from build123d import *

# Parameters (mm, degrees)
SKETCH1_R             = 11
BOSS_EXTRUDE1_DEPTH   = 3
SKETCH1_3_R           = 11
CUT_EXTRUDE1_DEPTH    = 1
SKETCH2_W             = 3
SKETCH2_H             = 6
BOSS_EXTRUDE2_DEPTH   = 3
BOSS_EXTRUDE2_2_DEPTH = 3
SKETCH2_H_2           = 5.08
BOSS_EXTRUDE2_3_DEPTH = 3
BOSS_EXTRUDE2_4_DEPTH = 3
BOSS_EXTRUDE2_5_DEPTH = 3
SKETCH3_W             = 3
SKETCH3_H             = 3
CUT_EXTRUDE2_DEPTH    = 3


with BuildPart() as part:
    # Sketch1 → Boss-Extrude1 (new body)
    with BuildSketch(Plane.XY):
        Polygon((-15, -15), (-35, -26.54), (-35, 26.54), (-15, 15), (15, 15), (15, -15), align=None)
        Circle(SKETCH1_R, mode=Mode.SUBTRACT)
        Circle(SKETCH1_R)
    extrude(amount=BOSS_EXTRUDE1_DEPTH)

    # Sketch1_3 → Cut-Extrude1 (cut)
    with BuildSketch(Plane.XY):
        Circle(SKETCH1_3_R)
    extrude(amount=CUT_EXTRUDE1_DEPTH, mode=Mode.SUBTRACT)

    # Sketch3 → Cut-Extrude2 (cut)
    with BuildSketch(Plane(origin=(0, 0, 0), x_dir=(-1, 0, 0), z_dir=(0, 0, -1))):
        with Locations((22, 0)):
            Rectangle(SKETCH3_W, SKETCH3_H)
        with Locations((16.5, 0)):
            Rectangle(SKETCH3_W, SKETCH3_H)
        with Locations((27.5, 0)):
            Rectangle(SKETCH3_W, SKETCH3_H)
        with Locations((33, 0)):
            Rectangle(SKETCH3_W, SKETCH3_H)
    extrude(amount=-CUT_EXTRUDE2_DEPTH, mode=Mode.SUBTRACT)


with BuildPart() as body_2:
    # Sketch2 → Boss-Extrude2 (new body)
    with BuildSketch(Plane(origin=(0, 0, 0), x_dir=(-1, 0, 0), z_dir=(0, 0, -1))):
        with Locations((36.5, -23.54)):
            Rectangle(SKETCH2_W, SKETCH2_H)
    extrude(amount=-BOSS_EXTRUDE2_DEPTH)


with BuildPart() as body_3:
    # Sketch2 → Boss-Extrude2 2 (new body)
    with BuildSketch(Plane(origin=(0, 0, 0), x_dir=(-1, 0, 0), z_dir=(0, 0, -1))):
        with Locations((36.5, -11.54)):
            Rectangle(SKETCH2_W, SKETCH2_H)
    extrude(amount=-BOSS_EXTRUDE2_2_DEPTH)


with BuildPart() as body_4:
    # Sketch2 → Boss-Extrude2 3 (new body)
    with BuildSketch(Plane(origin=(0, 0, 0), x_dir=(-1, 0, 0), z_dir=(0, 0, -1))):
        with Locations((36.5, 0)):
            Rectangle(SKETCH2_W, SKETCH2_H_2)
    extrude(amount=-BOSS_EXTRUDE2_3_DEPTH)


with BuildPart() as body_5:
    # Sketch2 → Boss-Extrude2 4 (new body)
    with BuildSketch(Plane(origin=(0, 0, 0), x_dir=(-1, 0, 0), z_dir=(0, 0, -1))):
        with Locations((36.5, 11.54)):
            Rectangle(SKETCH2_W, SKETCH2_H)
    extrude(amount=-BOSS_EXTRUDE2_4_DEPTH)


with BuildPart() as body_6:
    # Sketch2 → Boss-Extrude2 5 (new body)
    with BuildSketch(Plane(origin=(0, 0, 0), x_dir=(-1, 0, 0), z_dir=(0, 0, -1))):
        with Locations((36.5, 23.54)):
            Rectangle(SKETCH2_W, SKETCH2_H)
    extrude(amount=-BOSS_EXTRUDE2_5_DEPTH)


with BuildPart() as body_4_1:
    add(body_4.part)

    # Combine1: union body 2, body 5, part, body 6, body 3
    add(body_2.part)
    add(body_5.part)
    add(part.part)
    add(body_6.part)
    add(body_3.part)


solid = body_4_1.part
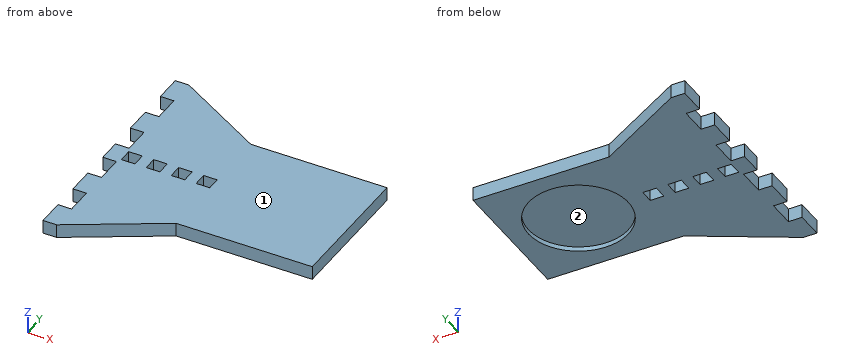
CAD build for the part. Positions are in the model's coordinates, mm. Face numbers are marked on the shaded views. Round coordinates to 2 decimals unless told otherwise and drop trailing zeros. Write each loop counter-clockwise with the first axis right and the second up, starting at its lowest first coordinate (ties: lowest second). Pieces come first, ordered by that corner, then holes. Notation, with made-up numbers: (-6.5, -22) -> (18.5, -22) arc R8 cw to (18.5, -17) -> close; hole circle Ø7 at (8.25, -9). An arc over 180 degrees is marked (long way). Answer as a JSON object with one key per item and string values.
(1) Band-saw the part on C-C, the plane z = 2.3. Count the separate pieces of the cut face and the enclosed holes in it, then the cut area to 3 significant figures.
Reported:
{"separate pieces": "1", "enclosed holes": "4", "area": "1,780 mm^2"}
(2) Probe probe 1 along Y at (x, z) = (0, 0.45); probe 2 along X at (y, z) = (-1, 0.8); probe 3 along Y at (x, z) = (12.5, 0.65). List the from-to ranges inside material, lowest first. Write a range as [from, to].
Reported:
{"probe 1": "y = [-15, -11], [11, 15]", "probe 2": "x = [-38, -34.5], [-31.5, -29], [-26, -23.5], [-20.5, -18], [-15, -10.95], [10.95, 15]", "probe 3": "y = [-15, 15]"}
(3) Pin check, flat tips, straight feed: P1, Ø1.5, axis at x = -16, z = 1.5, coming from the +Y side; P2, Ø1.5, axis at y = 6, z = 1, coming from the -X side; P3, Ø0.9, axis at x = -33.5, z = 1, coming from the -Y side. Stop position of each tip, or through.
Reported:
{"P1": "stops at y = 16.01", "P2": "stops at x = -35", "P3": "stops at y = -25.93"}
(4) Band-saw the part on A-A, the plane y = 0. List the corners of the cut face in (x, z), then the cut area to 3 significant figures.
Reported:
{"outline": "(-38, 0) -> (-34.5, 0) -> (-34.5, 3) -> (-38, 3) -> close; (-31.5, 0) -> (-29, 0) -> (-29, 3) -> (-31.5, 3) -> close; (-26, 0) -> (-23.5, 0) -> (-23.5, 3) -> (-26, 3) -> close; (-20.5, 0) -> (-18, 0) -> (-18, 3) -> (-20.5, 3) -> close; (-15, 0) -> (-11, 0) -> (-11, 1) -> (11, 1) -> (11, 0) -> (15, 0) -> (15, 3) -> (-15, 3) -> close", "area": "101 mm^2"}
(5) Band-saw the part on D-D, the plane x = -24.5. List the corners of the cut face in (y, z).
Reported:
{"outline": "(-20.48, 0) -> (20.48, 0) -> (20.48, 3) -> (-20.48, 3) -> close"}
(6) Two-plate mould, pull along X, no slides. Class the marked faces 1 and 2: +X half, -X half, draft (parallel to the pull), parting line (faces both ways), or undercut.
Reported:
{"face 1": "draft", "face 2": "undercut"}
(7) Band-saw the part on B-B, the plane x = 0. List the corners of the cut face in (y, z).
Reported:
{"outline": "(-15, 0) -> (-11, 0) -> (-11, 1) -> (11, 1) -> (11, 0) -> (15, 0) -> (15, 3) -> (-15, 3) -> close"}
